from build123d import *

# Parameters (mm, degrees)
SKETCH1_R           = 9
SKETCH1_R_2         = 7.5
BOSS_EXTRUDE1_DEPTH = 530
SKETCH2_R           = 17.5
SKETCH2_R_2         = 7.5
BOSS_EXTRUDE2_DEPTH = 10
BOSS_EXTRUDE3_START = -20
SKETCH3_R           = 17.5
SKETCH3_R_2         = 7.5
BOSS_EXTRUDE3_DEPTH = 20
CUT_EXTRUDE1_START  = -10
SKETCH4_R           = 17.5
SKETCH4_R_2         = 13.5
CUT_EXTRUDE1_DEPTH  = 10


with BuildPart() as part:
    # Sketch1 → Boss-Extrude1 (new body)
    with BuildSketch(Plane.XY):
        Circle(SKETCH1_R)
        Circle(SKETCH1_R_2, mode=Mode.SUBTRACT)
    extrude(amount=BOSS_EXTRUDE1_DEPTH)

    # Sketch2 → Boss-Extrude2 (add)
    with BuildSketch(Plane(origin=(0, 0, 0), x_dir=(-1, 0, 0), z_dir=(0, 0, -1))):
        Circle(SKETCH2_R)
        with Locations(Location((0, 0, 0), (0, 0, 180))):
            Circle(SKETCH2_R_2, mode=Mode.SUBTRACT)
    extrude(amount=-BOSS_EXTRUDE2_DEPTH)

    # Sketch3 → Boss-Extrude3 (add)
    with BuildSketch(Plane.XY.offset(530).offset(BOSS_EXTRUDE3_START)):
        with Locations(Location((0, 0, 0), (0, 0, 180))):
            Circle(SKETCH3_R)
        Circle(SKETCH3_R_2, mode=Mode.SUBTRACT)
    extrude(amount=BOSS_EXTRUDE3_DEPTH)

    # Sketch4 → Cut-Extrude1 (cut)
    with BuildSketch(Plane.XY.offset(530).offset(CUT_EXTRUDE1_START)):
        Circle(SKETCH4_R)
        Circle(SKETCH4_R_2, mode=Mode.SUBTRACT)
    extrude(amount=CUT_EXTRUDE1_DEPTH, mode=Mode.SUBTRACT)


solid = part.part
Here's how the part is built. I have some questions about the finished solid (model axes, mm). A direction names the side the tool comes from. Round coordinates to 2 decimals unless told otherwise and drop trailing zeros. Write each loop counter-clockwise with the first axis right and the second up, starting at its lowest first coordinate (ties: lowest second). Pieces come first, ordered by that corner, then holes. Notation, with made-up numbers: (20, 71.5) -> (25, 71.5) arc R29 cw to (25, 96.5) -> close; hole circle Ø3 at (75.5, -24). An arc over 180 degrees is marked (long way). One line per item, written item: value.
1) I'm going to push flat-ended pins straight in: pin 1 Ø10 at (y, z) = (-3, 174.5) entering from -X; pin 2 Ø3 at (x, z) = (-6.5, 300.5) entering from -Y; pin 3 Ø12 at (x, z) = (-12.5, 115.5) entering from -Y. Where does each tip first touch, or does it pass through?
Filled sheet:
pin 1: stops at x = -9
pin 2: stops at y = -7.48
pin 3: stops at y = -6.22
2) If I drill on line 1 (Z direction, x = -7.5, y = 11); line 2 (Y direction, x = -1, z = 321); line 3 (Y direction, x = 0, z = 270.5), over which ranges is the centre line in solid material (lowest first)? Write a range as [from, to].
Filled sheet:
line 1: z = [0, 10], [510, 530]
line 2: y = [-8.94, -7.43], [7.43, 8.94]
line 3: y = [-9, -7.5], [7.5, 9]
3) For faces 1 (the face through (-8, -8, 10)), 2 (the face through (3.794, 17.084, 514.93)), which set-ups out of +Z, -Z, +X, -X, +Y, -Y let a thin tool reach every point of the face, with its end or its side?
Filled sheet:
face 1: none
face 2: +Z, -Z
4) Suppose I cut it at C-C on z = 401. List the corners of the cut face in (x, y) for me.
Filled sheet:
outline: circle Ø18 at (0, 0); hole circle Ø15 at (0, 0)
5) Suppose I cut it at A-A on y = 0. List the corners of the cut face in (x, z) for me, plus the area to 3 significant figures.
Filled sheet:
outline: (-17.5, 0) -> (-7.5, 0) -> (-7.5, 530) -> (-13.5, 530) -> (-13.5, 520) -> (-17.5, 520) -> (-17.5, 510) -> (-9, 510) -> (-9, 10) -> (-17.5, 10) -> close; (7.5, 0) -> (17.5, 0) -> (17.5, 10) -> (9, 10) -> (9, 510) -> (17.5, 510) -> (17.5, 520) -> (13.5, 520) -> (13.5, 530) -> (7.5, 530) -> close
area: 2,020 mm2
6) We'd pull the mould along Y, two halves only. Please class faces 3 (the face through (-2.93, -13.18, 524.93)), 4 (the face through (-7.493, 0.33, 261.29)), 5 (the face through (9, -10.3, 520)): released by +Y, released by -Y, zero draft, split by the parting line, or undercut.
Filled sheet:
face 3: split by the parting line
face 4: undercut
face 5: zero draft
